Build history of the part. All positions in model axes, mm. Face numbers are marked on the shaded views. A direction names the side the tool comes from. Give positions to 0.01 mm unless a question says otherwise; leave off trailing zeros. Loops run counter-clockwise (first coordinate to the right, second up) from the corner with the lowest first, then second, coordinate; pieces in that order, holes last.
1) Flat gauge pins, fed straight in: P1, Ø12, axis at x = 18, z = 27, coming from the +Y side; P2, Ø5, axis at x = -18.5, z = 12, coming from the -Y side; P3, Ø5, axis at x = -0.5, y = -57, coming from the +Z side; P4, Ø12, axis at x = 28, z = 4.5, coming from the -Y side. Where does each tip first touch, or does it go through?
2) 3-axis set-ups, long thin cutter, end or side, ignore diameter. For the marked faces 1, 2 and 3: which of +Z, -Z, +X, -X, +Y, -Y reach the whole face in a straight line?
3) Two-plate mould, pull along X, no slides. Class the marked faces 4, 5, 6 and 7: +X half, -X half, draft (parallel to the pull), parting line (faces both ways), or undercut.
4) Wall check: line 1 (Z direction, x = 1, y = -48); line 2 (X direction, y = -45.5, z = -7); line 3 (Y direction, x = -25, z = 28.5). Give the ranges that are in metal, low to high.
5) Band-saw the part on A-A on y = -35. List the corners of the cut face in (x, z), then the cut area to 3 significant figures.
```python
from build123d import *

# Parameters (mm, degrees)
F0_W     = 80
F0_H     = 70
F1_DEPTH = 50
F2_R     = 23.84042
F3_DEPTH = 25.4
F4_R     = 5.08
F5_R     = 20.32
F6_W     = 12.7
F6_H     = 16.662312
F7_DEPTH = 75.4


with BuildPart() as f1:
    # F0 (on Front) → F1 (new body)
    with BuildSketch(Plane.XZ):
        Rectangle(F0_W, F0_H)
    extrude(amount=F1_DEPTH)

    # F2 (on face) → F3 (join)
    with BuildSketch(Plane.XZ.offset(50)):
        Circle(F2_R)
    extrude(amount=F3_DEPTH)

    # F4
    f4_edges = [f1.edges().sort_by_distance(p)[0] for p in [
        (40, -25, 35),
        (40, -25, -35),
        (-40, -25, 35),
        (-40, -25, -35),
    ]]
    fillet(f4_edges, radius=F4_R)

    # F5
    f5_edges = [f1.edges().sort_by_distance(p)[0] for p in [
        (-23.84042, -75.4, 0),
    ]]
    fillet(f5_edges, radius=F5_R)

    # F6 (on face) → F7 (cut, through all)
    with BuildSketch(Plane.XZ.offset(75.4)):
        Rectangle(F6_W, F6_H)
    extrude(amount=-F7_DEPTH, mode=Mode.SUBTRACT)


solid = f1.part
```
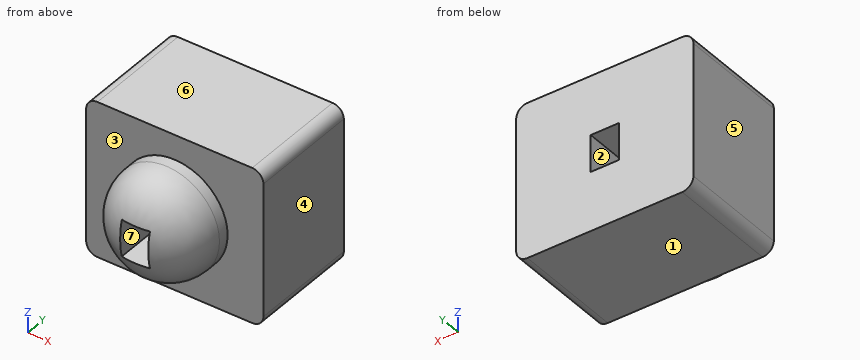
Findings below:
1. P1: stops at y = 0
1. P2: stops at y = -67.57
1. P3: stops at z = 23.84
1. P4: stops at y = -62.7
2. face 1: -Z, +X, -X, +Y, -Y
2. face 2: +Y, -Y
2. face 3: -Y
3. face 4: +X half
3. face 5: -X half
3. face 6: draft
3. face 7: undercut
4. line 1: z = -35 to -8.33, 8.33 to 35
4. line 2: x = -40 to -6.35, 6.35 to 40
4. line 3: y = -50 to 0
5. outline: (-40, -29.92) arc R5.08 ccw to (-34.92, -35) - (34.92, -35) arc R5.08 ccw to (40, -29.92) - (40, 29.92) arc R5.08 ccw to (34.92, 35) - (-34.92, 35) arc R5.08 ccw to (-40, 29.92) - close; hole (-6.35, -8.33) - (6.35, -8.33) - (6.35, 8.33) - (-6.35, 8.33) - close
5. area: 5,370 mm2
